```python
from build123d import *

# Parameters (mm, degrees)
SKETCH1_R           = 1.5
SKETCH1_R_2         = 4.8
SKETCH1_R_3         = 4
BOSS_EXTRUDE1_DEPTH = 4
BOSS_EXTRUDE4_DEPTH = 4
SKETCH1_9_R         = 1.5
SKETCH1_9_R_2       = 40
SKETCH1_9_R_3       = 11
BOSS_EXTRUDE5_DEPTH = 4
SKETCH1_14_R        = 4
SKETCH1_14_R_2      = 3.85
BOSS_EXTRUDE6_DEPTH = 4
SKETCH1_15_R        = 4
SKETCH1_15_R_2      = 3.85
BOSS_EXTRUDE7_DEPTH = 4


with BuildPart() as part:
    # Sketch1 → Boss-Extrude1 (new body)
    with BuildSketch(Plane.XY):
        Polygon((-125, -100), (150, -100), (150, 100), (-125, 100), (-150, 0), align=None)
        with Locations((-100, -83.333333333)):
            Circle(SKETCH1_R, mode=Mode.SUBTRACT)
        with BuildLine():
            ThreePointArc((-28.85, 11.97315075), (-8.649816618, -5.22350704), (-0.090081146, -30.333333333))
            ThreePointArc((-0.090081146, -30.333333333), (-0.02252536, -31.832657268), (0, -33.333333333))
            ThreePointArc((0, -33.333333333), (-0.02252536, -34.834009399), (-0.090081146, -36.333333333))
            ThreePointArc((-0.090081146, -36.333333333), (-8.649816618, -61.443159627), (-28.85, -78.639817417))
            ThreePointArc((-28.85, -78.639817417), (-50, -83.333333333), (-71.15, -78.639817417))
            ThreePointArc((-71.15, -78.639817417), (-91.350183382, -61.443159627), (-99.909918854, -36.333333333))
            ThreePointArc((-99.909918854, -36.333333333), (-100, -33.333333333), (-99.909918854, -30.333333333))
            ThreePointArc((-99.909918854, -30.333333333), (-91.350183382, -5.22350704), (-71.15, 11.97315075))
            ThreePointArc((-71.15, 11.97315075), (-50, 16.666666667), (-28.85, 11.97315075))
        make_face(mode=Mode.SUBTRACT)
        with Locations((0, -83.333333333)):
            Circle(SKETCH1_R, mode=Mode.SUBTRACT)
        with Locations((107.142857143, -71.428571429)):
            Circle(SKETCH1_R_2, mode=Mode.SUBTRACT)
        with Locations((-100, 16.666666667)):
            Circle(SKETCH1_R, mode=Mode.SUBTRACT)
        with Locations((-107.142857143, 71.428571429)):
            Circle(SKETCH1_R_2, mode=Mode.SUBTRACT)
        with Locations((21.832408692, 6.152026506)):
            Circle(SKETCH1_R, mode=Mode.SUBTRACT)
        with Locations((0, 16.666666667)):
            Circle(SKETCH1_R, mode=Mode.SUBTRACT)
        with Locations((37.332408692, 21.652026506)):
            Circle(SKETCH1_R_3, mode=Mode.SUBTRACT)
        with Locations((52.832408692, 6.152026506)):
            Circle(SKETCH1_R, mode=Mode.SUBTRACT)
        with Locations((21.832408692, 37.152026506)):
            Circle(SKETCH1_R, mode=Mode.SUBTRACT)
        with Locations((52.832408692, 37.152026506)):
            Circle(SKETCH1_R, mode=Mode.SUBTRACT)
        with Locations((107.142857143, 71.428571429)):
            Circle(SKETCH1_R_2, mode=Mode.SUBTRACT)
    extrude(amount=BOSS_EXTRUDE1_DEPTH)

    # Sketch1_8 → Boss-Extrude4 (add)
    with BuildSketch(Plane.XY):
        with BuildLine():
            Line((-71.15, 10.312141804), (-71.15, 11.97315075))
            ThreePointArc((-71.15, 11.97315075), (-91.350183382, -5.22350704), (-99.909918854, -30.333333333))
            Line((-99.909918854, -30.333333333), (-98.5, -33.333333333))
            ThreePointArc((-98.5, -33.333333333), (-98.476776333, -31.832614732), (-98.407127574, -30.333333333))
            ThreePointArc((-98.407127574, -30.333333333), (-90.281039726, -6.320598585), (-71.15, 10.312141804))
        make_face()
        with BuildLine():
            Line((-98.5, -33.333333333), (-99.909918854, -30.333333333))
            ThreePointArc((-99.909918854, -30.333333333), (-100, -33.333333333), (-99.909918854, -36.333333333))
            Line((-99.909918854, -36.333333333), (-98.5, -33.333333333))
        make_face()
        with BuildLine():
            ThreePointArc((-98.5, -33.333333333), (-91.097597253, -59.086731167), (-71.15, -76.978808471))
            Line((-71.15, -76.978808471), (-71.15, -67.284437881))
            ThreePointArc((-71.15, -67.284437881), (-90, -33.333333333), (-71.15, 0.617771214))
            Line((-71.15, 0.617771214), (-71.15, 10.312141804))
            ThreePointArc((-71.15, 10.312141804), (-90.281039726, -6.320598585), (-98.407127574, -30.333333333))
            ThreePointArc((-98.407127574, -30.333333333), (-98.476776333, -31.832614732), (-98.5, -33.333333333))
        make_face()
        with BuildLine():
            Line((-71.15, -78.639817417), (-71.15, -76.978808471))
            ThreePointArc((-71.15, -76.978808471), (-91.097597253, -59.086731167), (-98.5, -33.333333333))
            Line((-98.5, -33.333333333), (-99.909918854, -36.333333333))
            ThreePointArc((-99.909918854, -36.333333333), (-91.350183382, -61.443159627), (-71.15, -78.639817417))
        make_face()
        with BuildLine():
            Line((-1.5, -33.333333333), (-0.090081146, -30.333333333))
            ThreePointArc((-0.090081146, -30.333333333), (-8.649816618, -5.22350704), (-28.85, 11.97315075))
            Line((-28.85, 11.97315075), (-28.85, 10.312141804))
            ThreePointArc((-28.85, 10.312141804), (-9.718960274, -6.320598585), (-1.592872426, -30.333333333))
            ThreePointArc((-1.592872426, -30.333333333), (-1.523223667, -31.832614732), (-1.5, -33.333333333))
        make_face()
        with BuildLine():
            ThreePointArc((-28.85, -76.978808471), (-8.902402747, -59.086731167), (-1.5, -33.333333333))
            ThreePointArc((-1.5, -33.333333333), (-1.523223667, -31.832614732), (-1.592872426, -30.333333333))
            ThreePointArc((-1.592872426, -30.333333333), (-9.718960274, -6.320598585), (-28.85, 10.312141804))
            Line((-28.85, 10.312141804), (-28.85, 0.617771214))
            ThreePointArc((-28.85, 0.617771214), (-15.0285831, -13.916845494), (-10, -33.333333333))
            ThreePointArc((-10, -33.333333333), (-15.0285831, -52.749821172), (-28.85, -67.284437881))
            Line((-28.85, -67.284437881), (-28.85, -76.978808471))
        make_face()
        with BuildLine():
            ThreePointArc((0, -33.333333333), (-0.02252536, -31.832657268), (-0.090081146, -30.333333333))
            Line((-0.090081146, -30.333333333), (-1.5, -33.333333333))
            Line((-1.5, -33.333333333), (-0.090081146, -36.333333333))
            ThreePointArc((-0.090081146, -36.333333333), (-0.02252536, -34.834009399), (0, -33.333333333))
        make_face()
        with BuildLine():
            Line((-0.090081146, -36.333333333), (-1.5, -33.333333333))
            ThreePointArc((-1.5, -33.333333333), (-8.902402747, -59.086731167), (-28.85, -76.978808471))
            Line((-28.85, -76.978808471), (-28.85, -78.639817417))
            ThreePointArc((-28.85, -78.639817417), (-8.649816618, -61.443159627), (-0.090081146, -36.333333333))
        make_face()
    extrude(amount=BOSS_EXTRUDE4_DEPTH)

    # Sketch1_9 → Boss-Extrude5 (add)
    # profile 1 of 13: a face of its own
    with BuildSketch(Plane.XY):
        with BuildLine():
            Line((-28.85, 10.312141804), (-28.85, 11.97315075))
            ThreePointArc((-28.85, 11.97315075), (-50, 16.666666667), (-71.15, 11.97315075))
            Line((-71.15, 11.97315075), (-71.15, 10.312141804))
            ThreePointArc((-71.15, 10.312141804), (-50, 15.166666667), (-28.85, 10.312141804))
        make_face()
    # profile 2 of 13: a face of its own
    with BuildSketch(Plane.XY):
        with BuildLine():
            Line((-28.85, 0.617771214), (-28.85, 10.312141804))
            ThreePointArc((-28.85, 10.312141804), (-50, 15.166666667), (-71.15, 10.312141804))
            Line((-71.15, 10.312141804), (-71.15, 0.617771214))
            ThreePointArc((-71.15, 0.617771214), (-50, 6.666666667), (-28.85, 0.617771214))
        make_face()
    # profile 3 of 13: a face of its own
    with BuildSketch(Plane.XY):
        with Locations((0, 16.666666667)):
            Circle(SKETCH1_9_R)
    # profile 4 of 13: a face of its own
    with BuildSketch(Plane.XY):
        with Locations((-100, 16.666666667)):
            Circle(SKETCH1_9_R)
    # profile 5 of 13: a face of its own
    with BuildSketch(Plane.XY):
        with Locations((-100, -83.333333333)):
            Circle(SKETCH1_9_R)
    # profile 6 of 13: a face of its own
    with BuildSketch(Plane.XY):
        with Locations((0, -83.333333333)):
            Circle(SKETCH1_9_R)
    # profile 7 of 13: a face of its own
    with BuildSketch(Plane.XY):
        with BuildLine():
            Line((-28.85, -78.639817417), (-28.85, -76.978808471))
            ThreePointArc((-28.85, -76.978808471), (-50, -81.833333333), (-71.15, -76.978808471))
            Line((-71.15, -76.978808471), (-71.15, -78.639817417))
            ThreePointArc((-71.15, -78.639817417), (-50, -83.333333333), (-28.85, -78.639817417))
        make_face()
    # profile 8 of 13: a face of its own
    with BuildSketch(Plane.XY):
        with BuildLine():
            ThreePointArc((-71.15, -76.978808471), (-50, -81.833333333), (-28.85, -76.978808471))
            Line((-28.85, -76.978808471), (-28.85, -67.284437881))
            ThreePointArc((-28.85, -67.284437881), (-50, -73.333333333), (-71.15, -67.284437881))
            Line((-71.15, -67.284437881), (-71.15, -76.978808471))
        make_face()
    # profile 9 of 13: a face of its own
    with BuildSketch(Plane.XY):
        with Locations((-50, -33.333333333)):
            Circle(SKETCH1_9_R_2)
        with Locations((-50, -33.333333333)):
            Circle(SKETCH1_9_R_3, mode=Mode.SUBTRACT)
        with Locations((-65.5, -48.833333333)):
            Circle(SKETCH1_9_R, mode=Mode.SUBTRACT)
        with Locations((-34.5, -48.833333333)):
            Circle(SKETCH1_9_R, mode=Mode.SUBTRACT)
        with Locations((-34.5, -17.833333333)):
            Circle(SKETCH1_9_R, mode=Mode.SUBTRACT)
        with Locations((-65.5, -17.833333333)):
            Circle(SKETCH1_9_R, mode=Mode.SUBTRACT)
    # profile 10 of 13: a face of its own
    with BuildSketch(Plane.XY):
        with Locations((52.832408692, 37.152026506)):
            Circle(SKETCH1_9_R)
    # profile 11 of 13: a face of its own
    with BuildSketch(Plane.XY):
        with Locations((21.832408692, 37.152026506)):
            Circle(SKETCH1_9_R)
    # profile 12 of 13: a face of its own
    with BuildSketch(Plane.XY):
        with Locations((21.832408692, 6.152026506)):
            Circle(SKETCH1_9_R)
    # profile 13 of 13: a face of its own
    with BuildSketch(Plane.XY):
        with Locations((52.832408692, 6.152026506)):
            Circle(SKETCH1_9_R)
    extrude(amount=BOSS_EXTRUDE5_DEPTH)

    # Sketch1_14 → Boss-Extrude6 (add)
    with BuildSketch(Plane.XY):
        with Locations((37.332408692, 21.652026506)):
            Circle(SKETCH1_14_R)
        with Locations((37.332408692, 21.652026506)):
            Circle(SKETCH1_14_R_2, mode=Mode.SUBTRACT)
    extrude(amount=BOSS_EXTRUDE6_DEPTH)

    # Sketch1_15 → Boss-Extrude7 (add)
    with BuildSketch(Plane.XY):
        with Locations((37.332408692, 21.652026506)):
            Circle(SKETCH1_15_R)
        with Locations((37.332408692, 21.652026506)):
            Circle(SKETCH1_15_R_2, mode=Mode.SUBTRACT)
    extrude(amount=BOSS_EXTRUDE7_DEPTH)


solid = part.part
```
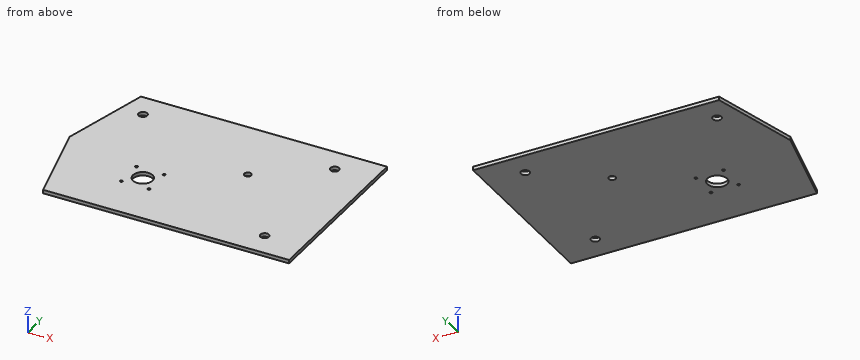
Can you work these out from the model? Positions are in its coordinate system, mm. Give positions to 0.01 mm unless a question says otherwise; leave off trailing zeros. Order: outer loops, then holes, each group sorted by start corner. A loop starts at its lowest first (then second) coordinate and runs counter-clockwise, first axis right, second up. Notation, with made-up numbers: M -22.75,21 L -1.75,21 A17 cw -1.75,40 Z; hole C 13,15 d8. An arc over 180 degrees is marked long. Write item = value, one per line. Start each with the question number.
Q1. I need wall thicknesses on probe 1 along Y at (x, z) = (-65.5, 1.65); probe 2 along Y at (x, z) = (-50, 1.7); probe 3 along X at (y, z) = (73.5, 2.2) (3 decimals). Which ranges of each line are inside material? Lowest first, please. Write a range as [from, to].
Q2. Suppose I cut it at B-B (z = 2.75). Count the separate pieces of the cut face and the enclosed holes in it, plus the area to 3 significant figures.
Q3. Will these pins go through, and if not, where does the flat tip stop? pin 1 Ø13 at (x, y) = (-50, -33.33) entering from -Z; pin 2 Ø1 at (y, z) = (75.5, 0.5) entering from -X; pin 3 Ø2 at (y, z) = (-58, 2) entering from -X.
Q4. Suppose I cut it at A-A (x = -50). Write out the boundary of the cut face in (y, z).
Q5. Suppose I cut it at C-C (y = 81). Write out the boundary of the cut face in (x, z).
Q6. Suppose I cut it at D-D (y = 41). Write out the boundary of the cut face in (x, z), plus the area to 3 significant figures.
Check result:
q1.probe_1 = [-100, -50.33], [-47.33, -19.33], [-16.33, 100]
q1.probe_2 = [-100, -44.33], [-22.33, 100]
q1.probe_3 = [-131.625, -111.473], [-102.813, 102.813], [111.473, 150]
q2.separate_pieces = 1
q2.enclosed_holes = 9
q2.area = 56,800 mm2
q3.pin_1 = through
q3.pin_2 = -131.25
q3.pin_3 = -135.75
q4.outline = M -100,0 L -44.33,0 L -44.33,4 L -100,4 Z; M -22.33,0 L 100,0 L 100,4 L -22.33,4 Z
q5.outline = M -129.75,0 L 150,0 L 150,4 L -129.75,4 Z
q6.outline = M -139.75,0 L 150,0 L 150,4 L -139.75,4 Z
q6.area = 1,160 mm2
